```python
from build123d import *

# Parameters (mm, degrees)
BOSS_EXTRUDE1_DEPTH = 2.54
SKETCH5_W           = 3.175
SKETCH5_H           = 19.05
CUT_EXTRUDE1_DEPTH  = 3.175
SKETCH6_R           = 27.938087672
CUT_EXTRUDE2_DEPTH  = 3.175


with BuildPart() as part:
    # Sketch2 → Boss-Extrude1 (new body)
    with BuildSketch(Plane.XY):
        with BuildLine():
            ThreePointArc((0, -200.025), (200.025, 0), (0, 200.025))
            ThreePointArc((0, 200.025), (-200.025, 0), (0, -200.025))
        make_face()
        with BuildLine():
            ThreePointArc((-73.279, -107.95), (-69.85, -104.521), (-66.421, -107.95))
            Line((-66.421, -107.95), (-66.421, -120.65))
            ThreePointArc((-66.421, -120.65), (-69.85, -124.079), (-73.279, -120.65))
            Line((-73.279, -120.65), (-73.279, -107.95))
        make_face(mode=Mode.SUBTRACT)
        with BuildLine():
            ThreePointArc((-167.810051257, -95.021689383), (-165.911659461, -96.754918821), (-167.644888899, -98.653310617))
            ThreePointArc((-167.644888899, -98.653310617), (-169.543280695, -96.920081179), (-167.810051257, -95.021689383))
        make_face(mode=Mode.SUBTRACT)
        with BuildLine():
            ThreePointArc((-73.279, -82.55), (-69.85, -79.121), (-66.421, -82.55))
            Line((-66.421, -82.55), (-66.421, -95.25))
            ThreePointArc((-66.421, -95.25), (-69.85, -98.679), (-73.279, -95.25))
            Line((-73.279, -95.25), (-73.279, -82.55))
        make_face(mode=Mode.SUBTRACT)
        with BuildLine():
            ThreePointArc((-1.613828712, -192.83861209), (0.83638791, -192.061171288), (1.613828712, -194.51138791))
            ThreePointArc((1.613828712, -194.51138791), (-0.83638791, -195.288828712), (-1.613828712, -192.83861209))
        make_face(mode=Mode.SUBTRACT)
        with BuildLine():
            ThreePointArc((66.421, -107.95), (69.85, -104.521), (73.279, -107.95))
            Line((73.279, -107.95), (73.279, -120.65))
            ThreePointArc((73.279, -120.65), (69.85, -124.079), (66.421, -120.65))
            Line((66.421, -120.65), (66.421, -107.95))
        make_face(mode=Mode.SUBTRACT)
        with BuildLine():
            ThreePointArc((66.421, -82.55), (69.85, -79.121), (73.279, -82.55))
            Line((73.279, -82.55), (73.279, -95.25))
            ThreePointArc((73.279, -95.25), (69.85, -98.679), (66.421, -95.25))
            Line((66.421, -95.25), (66.421, -82.55))
        make_face(mode=Mode.SUBTRACT)
        with BuildLine():
            Line((-44.45, -154.092269675), (-44.45, -84.242269675))
            ThreePointArc((-44.45, -84.242269675), (-95.179383339, -3.667081567), (-50.8, 80.572467382))
            Line((-50.8, 80.572467382), (-50.8, 95.25))
            Line((-50.8, 95.25), (2.71e-07, 95.25))
            Line((2.71e-07, 95.25), (50.8, 95.25))
            Line((50.8, 95.25), (50.8, 80.572467382))
            ThreePointArc((50.8, 80.572467382), (83.400427157, 46.010121169), (95.25, 0))
            ThreePointArc((95.25, 0), (81.567226875, -49.186888497), (44.45, -84.242269675))
            Line((44.45, -84.242269675), (44.45, -154.092269675))
            Line((44.45, -154.092269675), (-44.45, -154.092269675))
        make_face(mode=Mode.SUBTRACT)
        with BuildLine():
            ThreePointArc((166.196222545, -97.816922707), (166.748047371, -95.306252467), (169.258717611, -95.858077293))
            ThreePointArc((169.258717611, -95.858077293), (168.706892785, -98.368747533), (166.196222545, -97.816922707))
        make_face(mode=Mode.SUBTRACT)
        with BuildLine():
            ThreePointArc((-166.196222545, 97.816922707), (-166.748047371, 95.306252467), (-169.258717611, 95.858077293))
            ThreePointArc((-169.258717611, 95.858077293), (-168.706892785, 98.368747533), (-166.196222545, 97.816922707))
        make_face(mode=Mode.SUBTRACT)
        with BuildLine():
            ThreePointArc((1.613828712, 192.83861209), (-0.83638791, 192.061171288), (-1.613828712, 194.51138791))
            ThreePointArc((-1.613828712, 194.51138791), (0.83638791, 195.288828712), (1.613828712, 192.83861209))
        make_face(mode=Mode.SUBTRACT)
        with BuildLine():
            ThreePointArc((167.810051257, 95.021689383), (165.911659461, 96.754918821), (167.644888899, 98.653310617))
            ThreePointArc((167.644888899, 98.653310617), (169.543280695, 96.920081179), (167.810051257, 95.021689383))
        make_face(mode=Mode.SUBTRACT)
    extrude(amount=BOSS_EXTRUDE1_DEPTH)

    # Sketch5 → Cut-Extrude1 (cut)
    with BuildSketch(Plane(origin=(0, 0, 0), x_dir=(-1, 0, 0), z_dir=(0, 0, -1))):
        with Locations((49.2125, 124.476608207)):
            Rectangle(SKETCH5_W, SKETCH5_H)
        with Locations((0, 126.364925979)):
            Rectangle(SKETCH5_W, SKETCH5_H)
        with Locations((-49.2125, 124.476608207)):
            Rectangle(SKETCH5_W, SKETCH5_H)
    extrude(amount=-CUT_EXTRUDE1_DEPTH, mode=Mode.SUBTRACT)

    # Sketch6 → Cut-Extrude2 (cut)
    with BuildSketch(Plane(origin=(0, 0, 0), x_dir=(-1, 0, 0), z_dir=(0, 0, -1))):
        with Locations((-152.4, 0)):
            Circle(SKETCH6_R)
        with Locations((-107.763073453, 107.763073453)):
            Circle(SKETCH6_R)
        with Locations((107.763073453, 107.763073453)):
            Circle(SKETCH6_R)
        with Locations((152.4, 0)):
            Circle(SKETCH6_R)
        with Locations((107.763073453, -107.763073453)):
            Circle(SKETCH6_R)
        with Locations((-107.763073453, -107.763073453)):
            Circle(SKETCH6_R)
    extrude(amount=-CUT_EXTRUDE2_DEPTH, mode=Mode.SUBTRACT)


solid = part.part
```
CAD build for the part. Positions are in the model's coordinates, mm. A direction names the side the tool comes from. Coordinates: 2 decimals unless noted, no trailing zeros. Order: outer loops, then holes, each group sorted by start corner. A loop starts at its lowest first (then second) coordinate and runs counter-clockwise, first axis right, second up. Notation, with made-up numbers: (24.25, 48.5) - (54.25, 48.5) arc R36 cw to (54.25, 87.5) - close; hole circle Ø9 at (68, 34.25). An arc over 180 degrees is marked (long way). Use a Markdown table: item, result. Add a question column.
(1) Saw through at B-B (y = -39.5). Give the cut face in (x, z), then the cut area to 3 significant figures.
(2) Saw through at D-D (z = 1.8). Count the separate pieces of the cut face and the enclosed holes in it, then the cut area to 3 significant figures.
(3) Saw through at C-C (x = -101.5). Give the cut face in (y, z), then the cut area to 3 significant figures.
(4) Flat gauge pins, fed straight in: pin 1 (0.8 mm diameter, centred on y = -133.5, z = 0.5, fed in from -X); pin 2 (1.5 mm diameter, centred on x = -66.5, z = 2, fed in from -Y); pin 3 (1.3 mm diameter, centred on y = -87, z = 1, fed in from -X). Where does each tip first touch, or does it go through?
(5) Drill centre lines: line 1 along X through (y, z) = (-1, 2.2); line 2 along Y through (x, z) = (88, 1.9); line 3 along X through (y, z) = (-112.5, 0.3). Where is each one in solid material? Low to high. Write a range as [from, to].
(6) Pull direction Y, two halves, no side cores. Call faces 1 (the face through (135.674, -106.535, 1.252)), 2 (the face through (86, -42, 2.54)), 3 (the face through (135.674, 108.991, 1.252)), 4 (the face through (195.27, -43.36, 1.25)): +Y half, -Y half, draft (parallel to the pull), parting line (faces both ways), or undercut.
(7) Which spindle directions (+Z, -Z, +X, -X, +Y, -Y) get a long thin tool onto all of the face, cutting with end or side? Do faces 5 (the face through (-95.115, -5.061, 1.252)), 6 (the face through (86, -42, 0)). Say none if no direction does.
(8) Saw through at A-A (x = -158.5). Give the cut face in (y, z), then the cut area to 3 significant figures.
Solved:
| question | item | result |
|---|---|---|
| 1 | outline | (-196.09, 0) - (-86.67, 0) - (-86.67, 2.54) - (-196.09, 2.54) - close; (86.67, 0) - (196.09, 0) - (196.09, 2.54) - (86.67, 2.54) - close |
| 1 | area | 556 mm² |
| 2 | separate pieces | 1 |
| 2 | enclosed holes | 20 |
| 2 | area | 75,700 mm² |
| 3 | outline | (-172.36, 0) - (-134.99, 0) - (-134.99, 2.54) - (-172.36, 2.54) - close; (-80.54, 0) - (80.54, 0) - (80.54, 2.54) - (-80.54, 2.54) - close; (134.99, 0) - (172.36, 0) - (172.36, 2.54) - (134.99, 2.54) - close |
| 3 | area | 599 mm² |
| 4 | pin 1 | stops at x = -149.31 |
| 4 | pin 2 | stops at y = -188.91 |
| 4 | pin 3 | stops at x = -180.43 |
| 5 | line 1 | x = [-200.02, -180.32], [-124.48, -95.24], [95.24, 124.48], [180.32, 200.02] |
| 5 | line 2 | y = [-179.63, -127.51], [-88.02, -36.45], [36.45, 88.02], [127.51, 179.63] |
| 5 | line 3 | x = [-165.39, -135.3], [-80.23, -73.28], [-66.42, -44.45], [44.45, 66.42], [73.28, 80.23], [135.3, 165.39] |
| 6 | face 1 | undercut |
| 6 | face 2 | draft |
| 6 | face 3 | undercut |
| 6 | face 4 | parting line |
| 7 | face 5 | +Z, -Z |
| 7 | face 6 | -Z, +X, -X, +Y, -Y |
| 8 | outline | (-122.02, 0) - (-27.26, 0) - (-27.26, 2.54) - (-122.02, 2.54) - close; (27.26, 0) - (122.02, 0) - (122.02, 2.54) - (27.26, 2.54) - close |
| 8 | area | 481 mm² |
